from build123d import *

# Parameters (mm, degrees)
SKETCH1_W                        = 160
SKETCH1_H                        = 142
ROOF_DEPTH                       = 3
SKETCH2_W                        = 150
SKETCH2_H                        = 3
FRONT_AND_REAR_WALLS_DEPTH       = 72
FILLET1_R                        = 5
FRONT_COVER_REINFORCEMENT_DEPTH  = 10
REAR_START                       = -10
REAR_COVER_REINFORCEMENT_DEPTH   = 10
SKETCH5_W                        = 19
SKETCH5_H                        = 8
DISPLAY_CABLE_PASSTHRU_CUT_DEPTH = 10
SKETCH6_R                        = 28
FAN_CUTOUTS_DEPTH                = 10


with BuildPart() as part:
    # Sketch1 → ROOF (new body)
    with BuildSketch(Plane(origin=(0, 0, 0), x_dir=(1, 0, 0), z_dir=(0, 1, 0))):
        with Locations((35, -39)):
            Rectangle(SKETCH1_W, SKETCH1_H)
    extrude(amount=ROOF_DEPTH)

    # Sketch2 → FRONT AND REAR WALLS (add)
    with BuildSketch(Plane(origin=(0, 0, 0), x_dir=(1, 0, 0), z_dir=(0, 1, 0))):
        with Locations((35, 30.5)):
            Rectangle(SKETCH2_W, SKETCH2_H)
        with Locations((35, -108.5)):
            Rectangle(SKETCH2_W, SKETCH2_H)
    extrude(amount=-FRONT_AND_REAR_WALLS_DEPTH)

    # Fillet1
    fillet1_edges = [part.edges().sort_by_distance(p)[0] for p in [
        (-40, -72, -30.5),
        (110, -72, -30.5),
        (-40, -72, 108.5),
        (110, -72, 108.5),
    ]]
    fillet(fillet1_edges, radius=FILLET1_R)

    # Sketch3 → FRONT COVER REINFORCEMENT (add)
    with BuildSketch(Plane.XY.offset(110)):
        with BuildLine():
            Line((110, -67), (110, 0))
            Line((110, 0), (107, 0))
            Line((107, 0), (107, -67))
            ThreePointArc((107, -67), (106.414213562, -68.414213562), (105, -69))
            Line((105, -69), (-35, -69))
            ThreePointArc((-35, -69), (-36.414213562, -68.414213562), (-37, -67))
            Line((-37, -67), (-37, 0))
            Line((-37, 0), (-40, 0))
            Line((-40, 0), (-40, -67))
            ThreePointArc((-40, -67), (-38.535533906, -70.535533906), (-35, -72))
            Line((-35, -72), (105, -72))
            ThreePointArc((105, -72), (108.535533906, -70.535533906), (110, -67))
        make_face()
    extrude(amount=-FRONT_COVER_REINFORCEMENT_DEPTH)

    # Sketch4 → REAR COVER REINFORCEMENT (add)
    with BuildSketch(Plane(origin=(0, 0, -32), x_dir=(-1, 0, 0), z_dir=(0, 0, -1)).offset(REAR_START)):
        with BuildLine():
            Line((-110, 0), (-110, -67))
            ThreePointArc((-110, -67), (-108.535533906, -70.535533906), (-105, -72))
            Line((-105, -72), (35, -72))
            ThreePointArc((35, -72), (38.535533906, -70.535533906), (40, -67))
            Line((40, -67), (40, 0))
            Line((40, 0), (37, 0))
            Line((37, 0), (37, -67))
            ThreePointArc((37, -67), (36.414213562, -68.414213562), (35, -69))
            Line((35, -69), (-105, -69))
            ThreePointArc((-105, -69), (-106.414213562, -68.414213562), (-107, -67))
            Line((-107, -67), (-107, 0))
            Line((-107, 0), (-110, 0))
        make_face()
    extrude(amount=REAR_COVER_REINFORCEMENT_DEPTH)

    # Sketch5 → DISPLAY CABLE PASSTHRU CUT (cut)
    with BuildSketch(Plane.XY.offset(110)):
        with Locations((100.5, -46)):
            Rectangle(SKETCH5_W, SKETCH5_H)
    extrude(amount=-DISPLAY_CABLE_PASSTHRU_CUT_DEPTH, mode=Mode.SUBTRACT)

    # Sketch6 → FAN CUTOUTS (cut)
    with BuildSketch(Plane.XY.offset(110)):
        with Locations((-5, -37)):
            Circle(SKETCH6_R)
        with Locations((58, -37)):
            Circle(SKETCH6_R)
    extrude(amount=-FAN_CUTOUTS_DEPTH, mode=Mode.SUBTRACT)


solid = part.part
The listing builds one solid part. Answer for the finished solid, in the listing's coordinates (mm). A direction names the side the tool comes from. Round coordinates to 2 decimals unless told otherwise and drop trailing zeros. Write each loop counter-clockwise with the first axis right and the second up, starting at its lowest first coordinate (ties: lowest second). Pieces come first, ordered by that corner, then holes. Notation, with made-up numbers: (65, 34.5) - (119, 34.5) arc R17 ccw to (119, 52.5) - close; hole circle Ø4 at (37, 87.25). An arc over 180 degrees is marked (long way). Use a Markdown table: item, result. Add a question column.
1. The part is cut by section B-B (x = 93). Write down the section's boundary in (y, z).
2. A tool of negligible diameter and unlimited length cuts with its end or side. For faces 4 (the face through (-40, -34, -27)), 5 (the face through (-11.07, -64.334, 108.521)), 6 (the face through (110, -21, 105)), 7 (the face through (-37, -34, 104)), from which of +Z, -Z, +X, -X, +Y, -Y can it reach the whole face along a straight path? Write none if from no direction.
3. Flat-ended cylindrical pins translate along their axes: P1, Ø3, axis at y = -44.5, z = 107, coming from the -X side; P2, Ø6, axis at x = 90.5, z = 51, coming from the -Y side; P3, Ø2, axis at y = -49.5, z = -27, coming from the +X side. Find the tip coordinate at first contact, or state that the pin passes through.
4. The part is cut by section A-A (y = -37). Write down the section's boundary in (x, z), and give its area (3 significant figures).
5. Consider line 1 (Z direction, x = 45, y = -62); line 2 (Y direction, x = -5, z = 108.85); line 3 (Z direction, x = -38, y = -8.5). Determine where each line is inside the solid, lowest interval first.
6. For a pull along Z with two mould halves and no side action, classify faces 1 (the face through (34, 0, 38)), 2 (the face through (-39, -70, 105)), 3 (the face through (34, -35, -32)) as +Z half, -Z half, draft (parallel to the pull), parting line (faces both ways), or undercut.
7. The part is cut by section D-D (z = 39.5). Write down the section's boundary in (x, y), and give its area (3 significant figures).
8. The part is cut by section C-C (x = -5). Write down the section's boundary in (y, z).
Reported:
| question | item | result |
|---|---|---|
| 1 | outline | (-72, -32) - (3, -32) - (3, 110) - (-42, 110) - (-42, 107) - (0, 107) - (0, -29) - (-69, -29) - (-69, -22) - (-72, -22) - close; (-72, 100) - (-69, 100) - (-69, 107) - (-50, 107) - (-50, 110) - (-72, 110) - close |
| 2 | face 4 | +Z, -Z, -X, -Y |
| 2 | face 5 | +Z |
| 2 | face 6 | +Z, -Z, +X, -Y |
| 2 | face 7 | none |
| 3 | P1 | x = -40 |
| 3 | P2 | y = 0 |
| 3 | P3 | x = 110 |
| 4 | outline | (-40, -32) - (110, -32) - (110, -22) - (107, -22) - (107, -29) - (-37, -29) - (-37, -22) - (-40, -22) - close; (-40, 100) - (-37, 100) - (-37, 107) - (-33, 107) - (-33, 110) - (-40, 110) - close; (23, 107) - (30, 107) - (30, 110) - (23, 110) - close; (86, 107) - (107, 107) - (107, 100) - (110, 100) - (110, 110) - (86, 110) - close |
| 4 | area | 648 mm^2 |
| 5 | line 1 | -32 to -29, 107 to 110 |
| 5 | line 2 | -72 to -65, -9 to 3 |
| 5 | line 3 | -32 to -22, 100 to 110 |
| 6 | face 1 | undercut |
| 6 | face 2 | draft |
| 6 | face 3 | -Z half |
| 7 | outline | (-45, 0) - (115, 0) - (115, 3) - (-45, 3) - close |
| 7 | area | 480 mm^2 |
| 8 | outline | (-72, -32) - (3, -32) - (3, 110) - (-9, 110) - (-9, 107) - (0, 107) - (0, -29) - (-69, -29) - (-69, -22) - (-72, -22) - close; (-72, 100) - (-69, 100) - (-69, 107) - (-65, 107) - (-65, 110) - (-72, 110) - close |
